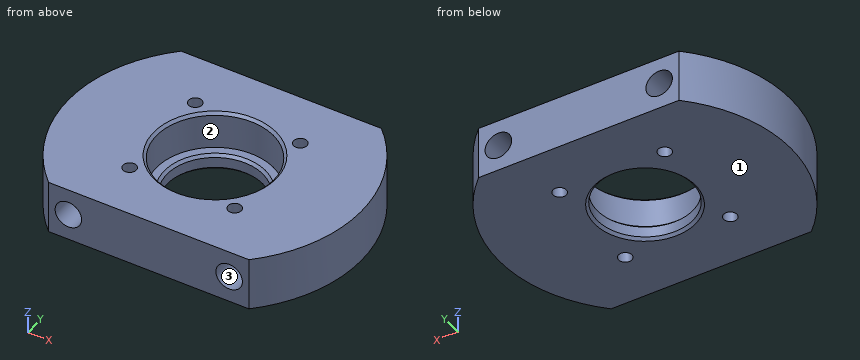
from build123d import *

# Parameters (mm, degrees)
ESQUISSE1_R             = 9
EXTRUSION1_DEPTH        = 10
ESQUISSE2_R             = 11
ENL_V_MAT_EXTRU_1_DEPTH = 7
CHANFREIN1_SIZE         = 0.5
TROU_TARAUD_M31_D       = 2.5
TROU_TARAUD_M31_DEPTH   = 10
ESQUISSE7_R             = 2.5
ENL_V_MAT_EXTRU_2_DEPTH = 41


with BuildPart() as part:
    # Esquisse1 → Extrusion1 (new body)
    with BuildSketch(Plane.XY):
        with BuildLine():
            Line((0, 0), (37.749172176, 0))
            ThreePointArc((37.749172176, 0), (46.374586088, 20), (37.749172176, 40))
            Line((37.749172176, 40), (0, 40))
            ThreePointArc((0, 40), (-8.625413912, 20), (0, 0))
        make_face()
        with Locations((18.874586088, 20)):
            Circle(ESQUISSE1_R, mode=Mode.SUBTRACT)
    extrude(amount=EXTRUSION1_DEPTH)

    # Esquisse2 → Enlèv. mat.-Extru.1 (cut)
    with BuildSketch(Plane.XY.offset(10)):
        with Locations((18.874586088, 20)):
            Circle(ESQUISSE2_R)
    extrude(amount=-ENL_V_MAT_EXTRU_1_DEPTH, mode=Mode.SUBTRACT)

    # Chanfrein1
    chanfrein1_edges = [part.edges().sort_by_distance(p)[0] for p in [
        (9.874586088, 20, 0),
        (9.874586088, 20, 3),
        (7.874586088, 20, 10),
    ]]
    chamfer(chanfrein1_edges, length=CHANFREIN1_SIZE)

    # Trou taraudé M31
    with Locations(Plane.XY.offset(10)):
        with Locations((28.774081025, 29.899494937), (8.975091152, 29.899494937), (8.975091152, 10.100505063), (28.774081025, 10.100505063)):
            Hole(TROU_TARAUD_M31_D / 2, depth=TROU_TARAUD_M31_DEPTH)

    # Esquisse7 → Enlèv. mat.-Extru.2 (cut, through all)
    with BuildSketch(Plane(origin=(0, 40, 0), x_dir=(1, 0, 0), z_dir=(0, 1, 0))):
        with Locations((3.725091152, -5)):
            Circle(ESQUISSE7_R)
        with Locations((34.024081025, -5)):
            Circle(ESQUISSE7_R)
    extrude(amount=-ENL_V_MAT_EXTRU_2_DEPTH, mode=Mode.SUBTRACT)


solid = part.part
Read the model definition and answer for the solid it produces. Units are mm, in the model's axes. Face numbers are marked on the shaded views. Round coordinates to 2 decimals unless told otherwise and drop trailing zeros. Loops run counter-clockwise (first coordinate to the right, second up) from the corner with the lowest first, then second, coordinate; pieces in that order, holes last.
Q1. Determine the mould class of the marked faces 1, 2 and 3 for opening direction Z: released by +Z, released by -Z, zero draft, split by the parting line, or undercut.
Q2. Section A-A on y = 20 is taken. Write down the section's boundary in (x, z), and give its area (3 significant figures).
Q3. Section D-D on y = 3.5 is taken. Write down the section's boundary in (x, z), and give its area (3 significant figures).
Q4. Each of these flat-tipped pins is pushed along its axis until it touches: pin 1 (3 mm diameter, centred on y = 21.5, z = 6, fed in from -X); pin 2 (1.5 mm diameter, centred on x = 28.77, y = 29.9, fed in from +Z). Where does it stop, or does it pass through?
Q5. Section B-B on z = 5 is taken. Write down the section's boundary in (x, y).
Q6. Section C-C on x = 35 is taken. Write down the section's boundary in (y, z), and give its area (3 significant figures).
Q7. Consider probe 1 along X at (y, z) = (11, 7.75); probe 2 along X at (y, z) = (20, 1.25); probe 3 along X at (y, z) = (21.5, 5). Determine where each line is inside the solid, lowest interval first.
Output:
1. face 1: released by -Z
1. face 2: zero draft
1. face 3: undercut
2. outline: (-8.63, 0) - (9.37, 0) - (9.87, 0.5) - (9.87, 2.5) - (9.37, 3) - (7.87, 3) - (7.87, 9.5) - (7.37, 10) - (-8.63, 10) - close; (27.87, 0.5) - (28.37, 0) - (46.37, 0) - (46.37, 10) - (30.37, 10) - (29.87, 9.5) - (29.87, 3) - (28.37, 3) - (27.87, 2.5) - close; hole circle Ø5 at (3.73, 5); hole circle Ø5 at (34.02, 5)
2. area: 302 mm2
3. outline: (-3.13, 0) - (40.87, 0) - (40.87, 10) - (-3.13, 10) - close; hole circle Ø5 at (3.73, 5); hole circle Ø5 at (34.02, 5)
3. area: 401 mm2
4. pin 1: stops at x = -8.63
4. pin 2: passes through
5. outline: (0, 0) - (1.23, 0) - (1.23, 40) - (0, 40) arc R27.5 ccw to start; (6.23, 0) - (31.52, 0) - (31.52, 40) - (6.23, 40) - close; (36.52, 0) - (37.75, 0) arc R27.5 ccw to (37.75, 40) - (36.52, 40) - close; hole circle Ø2.5 at (8.98, 10.1); hole circle Ø2.5 at (8.98, 29.9); hole circle Ø22 at (18.87, 20); hole circle Ø2.5 at (28.77, 10.1); hole circle Ø2.5 at (28.77, 29.9)
6. outline: (0, 0) - (40, 0) - (40, 2.7) - (0, 2.7) - close; (0, 7.3) - (40, 7.3) - (40, 10) - (0, 10) - close
6. area: 216 mm2
7. probe 1: x = -7.11 to 8.11, 9.84 to 12.55, 25.2 to 27.91, 29.64 to 44.86
7. probe 2: x = -8.63 to 9.87, 27.87 to 46.37
7. probe 3: x = -8.58 to 1.23, 6.23 to 7.98, 29.77 to 31.52, 36.52 to 46.33
